Can you work these out from the drawing? Everything is in mm from the part's minimum corner. Give positions to 0.01 mm unless a question says otherwise; leave off trailing zeros. Loops run counter-clockwise (first coordinate to the right, second up) from the corner with the lowest first, then second, coordinate; pieces in that order, holes last. Notation, with made-up numbers: (38.25, 14) -> (93.25, 14) arc R31 cw to (93.25, 49) -> close; hole circle Ø3 at (81.5, 67). An arc over 180 degrees is marked (long way). Write item = value, one per line. Start each with the question number.
1) I want a section at C-C (x = 55). List the corners of the cut face in (y, z) for me, and give its area (3 significant figures).
2) I want a section at A-A (z = 55). List the corners of the cut face in (x, y) for me.
3) I need wall thicknesses on probe 1 along Z at (x, y) = (54.5, 1.5); probe 2 along X at (y, z) = (1.85, 32.5). Which ranges of each line are inside material? Lowest first, please. Write a range as from..to.
4) I'm going to push flat-ended pins straight in: pin 1 Ø1 at (y, z) = (0.5, 82.5) entering from +X; pin 2 Ø1.5 at (y, z) = (2, 49) entering from -X; pin 3 Ø1 at (y, z) = (2, 77.5) entering from +X. Where does each tip first touch, or does it pass through?
5) I want a section at B-B (y = 2.35). Count the separate pieces of the cut face and the enclosed holes in it, and give its area (3 significant figures).
6) I want a section at D-D (x = 25.5). List the corners of the cut face in (y, z) for me.
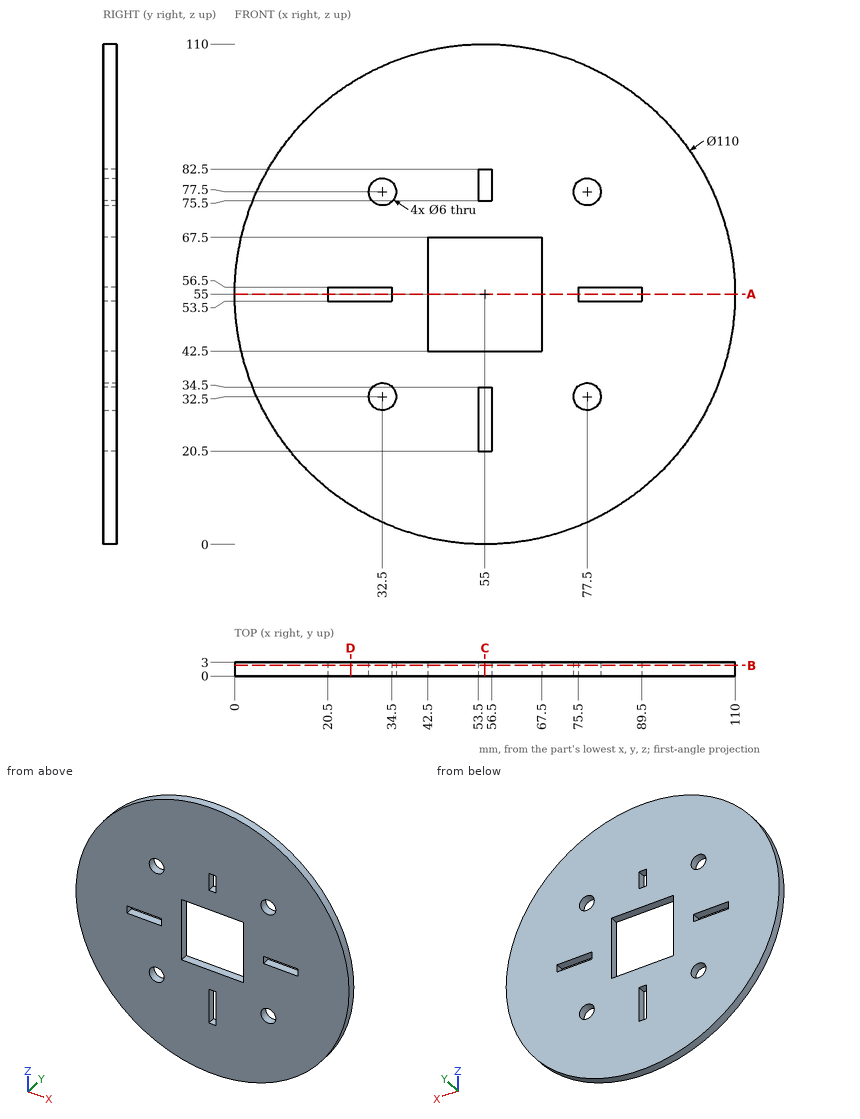
Answer list:
q1.outline = (0, 0) -> (3, 0) -> (3, 20.5) -> (0, 20.5) -> close; (0, 34.5) -> (3, 34.5) -> (3, 42.5) -> (0, 42.5) -> close; (0, 67.5) -> (3, 67.5) -> (3, 75.5) -> (0, 75.5) -> close; (0, 82.5) -> (3, 82.5) -> (3, 110) -> (0, 110) -> close
q1.area = 192 mm^2
q2.outline = (0, 0) -> (20.5, 0) -> (20.5, 3) -> (0, 3) -> close; (34.5, 0) -> (42.5, 0) -> (42.5, 3) -> (34.5, 3) -> close; (67.5, 0) -> (75.5, 0) -> (75.5, 3) -> (67.5, 3) -> close; (89.5, 0) -> (110, 0) -> (110, 3) -> (89.5, 3) -> close
q3.probe_1 = 0..20.5, 34.5..42.5, 67.5..75.5, 82.5..110
q3.probe_2 = 4.81..29.5, 35.5..53.5, 56.5..74.5, 80.5..105.19
q4.pin_1 = 102.92
q4.pin_2 = 0.25
q4.pin_3 = 105.41
q5.separate_pieces = 1
q5.enclosed_holes = 9
q5.area = 8,620 mm^2
q6.outline = (0, 8.58) -> (3, 8.58) -> (3, 53.5) -> (0, 53.5) -> close; (0, 56.5) -> (3, 56.5) -> (3, 101.42) -> (0, 101.42) -> close
